Geometry: final body of the model. Coordinates: model frame, mm. A direction names the side the tool comes from. Give positions to 0.01 mm unless a question says otherwise; leave off trailing zeros. Loops run counter-clockwise (first coordinate to the right, second up) from the corner with the lowest first, then second, coordinate; pieces in that order, holes last.
1. Draft query along Z for faces 3 (the face through (-63, 0, 32)), 4 (the face through (-32, 0, 34)), 5 (the face through (-21.5, 0.22, 4.93)). Return one class per face: +Z half, -Z half, draft (parallel to the pull), parting line (faces both ways), or undercut.
2. Section B-B, the plane y = 4.5. Output: boundary loops of the cut face in (x, z), then the cut area to 3 significant figures.
3. Section A-A, the plane x = 0. Output: boundary loops of the cut face in (y, z).
4. Material intervals for line 1 along Z through (x, y) = (0, -11.5); line 2 along Z through (x, y) = (-27, -14.5); line 3 along Y through (x, z) = (0, 20), sorted ascending.
5. Access query for faces 1 (the face through (-48.99, -11.85, 32.23)), 2 (the face through (-47, -3, 30.5)). Directions: +Z, -Z, +X, -X, +Y, -Y. A direction counts if a zero-diameter tool reaches every point of the face in a straight line with its end or side. Return the directions, or none.
6. First-contact query: P1, Ø10, axis at y = 4.5, z = 17.5, coming from the -X side; P2, Ø1.5, axis at y = 5, z = 28, coming from the +X side; P3, Ø1.5, axis at y = 7, z = 6.5, coming from the -X side. Flat tips, straight axial feed; report the tip coordinate or a pass-through.
7. Section D-D, the plane y = 13.5. Output: boundary loops of the cut face in (x, z), then the cut area to 3 significant figures.
8. Section C-C, the plane z = 32.5. Output: boundary loops of the cut face in (x, y), then the cut area to 3 significant figures.
from build123d import *

# Parameters (mm, degrees)
SKETCH_1_R          = 3
SKETCH_1_W          = 32
SKETCH_1_H          = 31.908510126
EXTRUDE_1_DEPTH     = 34
CUT_EXTRUDE_START   = -3.5
SKETCH_4_W          = 70
SKETCH_4_H          = 50
CUT_EXTRUDE_3_DEPTH = 27
FILLET_1_R          = 5
SKETCH_3_R          = 9
CUT_EXTRUDE_5_DEPTH = 35
SKETCH_8_R          = 4
CUT_EXTRUDE_6_DEPTH = 20
FILLET_2_R          = 5


with BuildPart() as part:
    # 草圖1 → 填料-伸長1 (new body)
    with BuildSketch(Plane.XY):
        with BuildLine():
            Line((-21.681969888, -15.954255063), (-21.681969888, 15.954255063))
            Line((-21.681969888, 15.954255063), (-75.189189189, 7.911120595))
            ThreePointArc((-75.189189189, 7.911120595), (-82, 0), (-75.189189189, -7.911120595))
            Line((-75.189189189, -7.911120595), (-21.681969888, -15.954255063))
        make_face()
        with Locations((-74, 0)):
            Circle(SKETCH_1_R, mode=Mode.SUBTRACT)
        with Locations((-60, 0)):
            Circle(SKETCH_1_R, mode=Mode.SUBTRACT)
        with Locations((-46, 0)):
            Circle(SKETCH_1_R, mode=Mode.SUBTRACT)
        with Locations((-5.681969888, 0)):
            Rectangle(SKETCH_1_W, SKETCH_1_H)
        with BuildLine():
            ThreePointArc((10.318030112, -15.954255063), (19, 0), (10.318030112, 15.954255063))
            Line((10.318030112, 15.954255063), (10.318030112, -15.954255063))
        make_face()
    extrude(amount=EXTRUDE_1_DEPTH)

    # 草圖4 → 除料-伸長3 (cut)
    with BuildSketch(Plane(origin=(0, 0, 0), x_dir=(-1, 0, 0), z_dir=(0, 0, -1)).offset(CUT_EXTRUDE_START)):
        with Locations((55, 0)):
            Rectangle(SKETCH_4_W, SKETCH_4_H)
    extrude(amount=-CUT_EXTRUDE_3_DEPTH, mode=Mode.SUBTRACT)

    # 圓角1
    fillet_1_edges = [part.edges().sort_by_distance(p)[0] for p in [
        (-20, 0, 3.5),
        (-20, 0, 30.5),
    ]]
    fillet(fillet_1_edges, radius=FILLET_1_R)

    # 草圖3 → 除料-伸長5 (cut, through all)
    with BuildSketch(Plane(origin=(0, 0, 0), x_dir=(-1, 0, 0), z_dir=(0, 0, -1))):
        Circle(SKETCH_3_R)
    extrude(amount=-CUT_EXTRUDE_5_DEPTH, mode=Mode.SUBTRACT)

    # 草圖8 → 除料-伸長6 (cut, symmetric)
    with BuildSketch(Plane(origin=(0, 0, 0), x_dir=(1, 0, 0), z_dir=(0, 1, 0))):
        with Locations((0, -25.75)):
            Circle(SKETCH_8_R)
        with Locations((0, -8.25)):
            Circle(SKETCH_8_R)
    extrude(amount=CUT_EXTRUDE_6_DEPTH, both=True, mode=Mode.SUBTRACT)

    # 圓角2
    fillet_2_edges = [part.edges().sort_by_distance(p)[0] for p in [
        (-21.681969888, -15.954255063, 2.379794385),
        (-21.681969888, -15.954255063, 31.620205615),
        (-21.681969888, 15.954255063, 2.379794385),
        (-21.681969888, 15.954255063, 31.620205615),
        (10.318030112, -15.954255063, 17),
        (10.318030112, 15.954255063, 17),
    ]]
    fillet(fillet_2_edges, radius=FILLET_2_R)


solid = part.part
Answers below:
1. face 3: draft
1. face 4: +Z half
1. face 5: undercut
2. outline: (-80.61, 0) - (-7.79, 0) - (-7.79, 34) - (-80.61, 34) - (-80.61, 30.5) - (-25, 30.5) arc R5 cw to (-20, 25.5) - (-20, 8.5) arc R5 cw to (-25, 3.5) - (-80.61, 3.5) - close; (7.79, 0) - (18.46, 0) - (18.46, 34) - (7.79, 34) - close
2. area: 1,210 mm2
3. outline: (-15.95, 0) - (-9, 0) - (-9, 4.25) - (-15.95, 4.25) - close; (-15.95, 12.25) - (-9, 12.25) - (-9, 21.75) - (-15.95, 21.75) - close; (-15.95, 29.75) - (-9, 29.75) - (-9, 34) - (-15.95, 34) - close; (9, 0) - (15.95, 0) - (15.95, 4.25) - (9, 4.25) - close; (9, 12.25) - (15.95, 12.25) - (15.95, 21.75) - (9, 21.75) - close; (9, 29.75) - (15.95, 29.75) - (15.95, 34) - (9, 34) - close
4. line 1: z = 0 to 4.25, 12.25 to 21.75, 29.75 to 34
4. line 2: z = 0 to 3.5, 30.5 to 34
4. line 3: y = -15.95 to -9, 9 to 15.95
5. face 1: +Z, -Z, -X, -Y
5. face 2: -X, +Y, -Y
6. P1: stops at x = -20
6. P2: stops at x = 18.52
6. P3: stops at x = -20.82
7. outline: (-38.01, 0) - (13.37, 0) - (13.37, 34) - (-38.01, 34) - (-38.01, 30.5) - (-25, 30.5) arc R5 cw to (-20, 25.5) - (-20, 8.5) arc R5 cw to (-25, 3.5) - (-38.01, 3.5) - close; hole circle Ø8 at (0, 8.25); hole circle Ø8 at (0, 25.75)
7. area: 1,170 mm2
8. outline: (-75.19, -7.91) - (-22.05, -15.9) arc R5 ccw to (-21.31, -15.95) - (8.72, -15.95) arc R5 ccw to (11.83, -14.87) arc R19 ccw to (11.83, 14.87) arc R5 ccw to (8.72, 15.95) - (-21.31, 15.95) arc R5 ccw to (-22.05, 15.9) - (-75.19, 7.91) arc R8 ccw to start; hole circle Ø6 at (-74, 0); hole circle Ø6 at (-60, 0); hole circle Ø6 at (-46, 0); hole circle Ø18 at (0, 0)
8. area: 2,230 mm2
